CAD build for the part. Positions are in the model's coordinates, mm. A direction names the side the tool comes from. Coordinates: 2 decimals unless noted, no trailing zeros. Write each loop counter-clockwise with the first axis right and the second up, starting at its lowest first coordinate (ties: lowest second). Pieces come first, ordered by that corner, then holes. Notation, with made-up numbers: (42, 54.25) - (94, 54.25) arc R34 cw to (94, 86.25) - close; hole circle Ø5 at (13.5, 66). An arc over 180 degrees is marked (long way). Answer in a Markdown table with one row per item. Add a question column.
Q1. Two-plate mould, pull along Z, no slides. Class faces 1 (the flat face through (0, -25, 40)), 2 (the flat face through (0, -33, 30)), 3 (the cylindrical face through (-0.28, -62.719, -37.594)), 4 (the flat face through (-9, 15, -8)): +Z half, -Z half, draft (parallel to the pull), parting line (faces both ways), or undercut.
Q2. Drill centre lines: line 1 along Z through (x, y) = (-11, -56); line 2 along Z through (x, y) = (0.5, 112); line 3 along Y through (x, z) = (-9.5, 9). Where is each one in solid material? Low to high. Write a range as from..to.
Q3. Pin check, flat tips, straight feed: pin 1 (12 mm diameter, centred on x = 0, y = 73.5, fed in from +Z); pin 2 (12 mm diameter, centred on x = -15, z = -30.5, fed in from +Y); pin 3 (10 mm diameter, centred on y = 87, z = -12, fed in from -X); pin 4 (2 mm diameter, centred on y = 60, z = 12.5, fed in from +X). Stop position of each tip, or through.
Q4. Band-saw the part on B-B (x = 0). List the corners of the cut face in (y, z).
Q5. Band-saw the part on C-C (z = 0). List the corners of the cut face in (x, y), and give its area (3 significant figures).
Q6. Band-saw the part on A-A (y = -6). List the corners of the cut face in (x, z), and give its area (3 significant figures).
Q7. 3-axis set-ups, long thin cutter, end or side, ignore diameter. For faces 5 (the cylindrical face through (-9.76, 81.55, -2.17)), 6 (the cylindrical face through (-5.09, -40.22, -0.42)), 7 (the flat face through (0, 0, 0)): which of +Z, -Z, +X, -X, +Y, -Y reach the whole face in a straight line?
Q8. Band-saw the part on D-D (z = -27). List the corners of the cut face in (x, y), and give its area (3 significant figures).
```python
from build123d import *

# Parameters (mm, degrees)
SKETCH_1_R           = 10
EXTRUDE_1_DEPTH      = 150
EXTRUDE_2_DEPTH      = 20
EXTRUDE_2_DEPTH_BACK = 20
EXTRUDE_3_REACH      = 168.733
SKETCH_3_R           = 11.024808504


with BuildPart() as part:
    # Sketch 1 → Extrude 1 (new body)
    with BuildSketch(Plane(origin=(0, 0, 0), x_dir=(1, 0, 0), z_dir=(0, 1, 0))):
        with Locations(Location((0, 0, 0), (0, 0, 270))):
            Circle(SKETCH_1_R)
    extrude(amount=EXTRUDE_1_DEPTH)

    # Sketch 2 → Extrude 2 (add, two sides: drawn at the far end of the back side and taken through both)
    with BuildSketch(Plane(origin=(0, 0, 0), x_dir=(0, 0, -1), z_dir=(1, 0, 0)).offset(-EXTRUDE_2_DEPTH_BACK)):
        with BuildLine():
            Line((-30, -65), (-30, 0))
            Line((-30, 0), (30, 0))
            Line((30, 0), (30, -65))
            Line((30, -65), (32, -65))
            ThreePointArc((32, -65), (37.656854249, -62.656854249), (40, -57))
            Line((40, -57), (40, 7))
            ThreePointArc((40, 7), (37.656854249, 12.656854249), (32, 15))
            Line((32, 15), (-32, 15))
            ThreePointArc((-32, 15), (-37.656854249, 12.656854249), (-40, 7))
            Line((-40, 7), (-40, -57))
            ThreePointArc((-40, -57), (-37.656854249, -62.656854249), (-32, -65))
            Line((-32, -65), (-30, -65))
        make_face()
    extrude(amount=EXTRUDE_2_DEPTH + EXTRUDE_2_DEPTH_BACK)

    # Sketch 3 → Extrude 3 (add, up to next)
    with BuildSketch(Plane.XY.offset(-30), mode=Mode.PRIVATE) as extrude_3_sk1:
        with Locations(Location((0, -50, 0), (0, 0, 180))):
            Circle(SKETCH_3_R)
    extrude_3_tool1 = extrude(extrude_3_sk1.sketch, amount=EXTRUDE_3_REACH, mode=Mode.PRIVATE) - part.part
    add(extrude_3_tool1.solids().sort_by_distance((0, -50, -30))[0])


solid = part.part
```
Checked values:
| question | item | result |
|---|---|---|
| 1 | face 1 | +Z half |
| 1 | face 2 | undercut |
| 1 | face 3 | -Z half |
| 1 | face 4 | draft |
| 2 | line 1 | z = -40..-30, 30..40 |
| 2 | line 2 | z = -9.99..9.99 |
| 2 | line 3 | y = -55.59..-44.41, 0..15 |
| 3 | pin 1 | stops at z = 10 |
| 3 | pin 2 | stops at y = 15 |
| 3 | pin 3 | stops at x = -7.14 |
| 3 | pin 4 | passes through |
| 4 | outline | (-65, -32) arc R8 ccw to (-57, -40) - (7, -40) arc R8 ccw to (15, -32) - (15, -10) - (150, -10) - (150, 10) - (15, 10) - (15, 32) arc R8 ccw to (7, 40) - (-57, 40) arc R8 ccw to (-65, 32) - (-65, 30) - (-61.02, 30) - (-61.02, -30) - (-65, -30) - close; hole (-38.98, -30) - (0, -30) - (0, 30) - (-38.98, 30) - close |
| 5 | outline | (-20, 0) - (20, 0) - (20, 15) - (10, 15) - (10, 150) - (-10, 150) - (-10, 15) - (-20, 15) - close; circle Ø22.05 at (0, -50) |
| 5 | area | 3,680 mm² |
| 6 | outline | (-20, -40) - (20, -40) - (20, -30) - (-20, -30) - close; (-20, 30) - (20, 30) - (20, 40) - (-20, 40) - close |
| 6 | area | 800 mm² |
| 7 | face 5 | +Y |
| 7 | face 6 | none |
| 7 | face 7 | +X, -X |
| 8 | outline | (-20, 0) - (20, 0) - (20, 15) - (-20, 15) - close; circle Ø22.05 at (0, -50) |
| 8 | area | 982 mm² |
